Could you check a few things on this model? Use its own coordinates, in mm. Face numbers are marked on the shaded views. A direction names the side the tool comes from. Give positions to 0.01 mm unless a question says otherwise; leave off trailing zeros. Order: outer loops, then holes, each group sorted by start corner. A loop starts at its lowest first (then second) coordinate and runs counter-clockwise, first axis right, second up. Notation, with made-up numbers: M 19.5,72 L 25.5,72 A23 cw 25.5,82 Z; hole C -36,11 d10. An arc over 180 degrees is marked long. Use a Markdown table: item, result. Add a question column.
Item 1: Suppose I cut it at B-B on x = 12.7. Write out the boundary of the cut face in (y, z).
Item 2: Suppose I cut it at D-D on y = -5.75. Write out the boundary of the cut face in (x, z).
Item 3: I'm going to push flat-ended pins straight in: pin 1 Ø12 at (y, z) = (-19, 3.5) entering from -X; pin 2 Ø4 at (x, z) = (33.5, 9) entering from -Y. Where does each tip first touch, or does it pass through?
Item 4: If I drill on L1, parallel to Z at x = 12.7, y = 2.1; L2, parallel to X at y = -9, z = 2; L3, parallel to Y at x = 43.5, z = 2.5, over which ranges is the centre line in solid material (lowest first)? Write a range as from..to.
Item 5: For the marked faces 1 and 2, which set-ups out of +Z, -Z, +X, -X, +Y, -Y let a thin tool reach every point of the face, with its end or its side?
Item 6: Suppose I cut it at A-A on z = 12.7. Write out the boundary of the cut face in (x, y), plus the area to 3 significant figures.
Item 7: Suppose I cut it at C-C on z = 24.25. Write out the boundary of the cut face in (x, y).
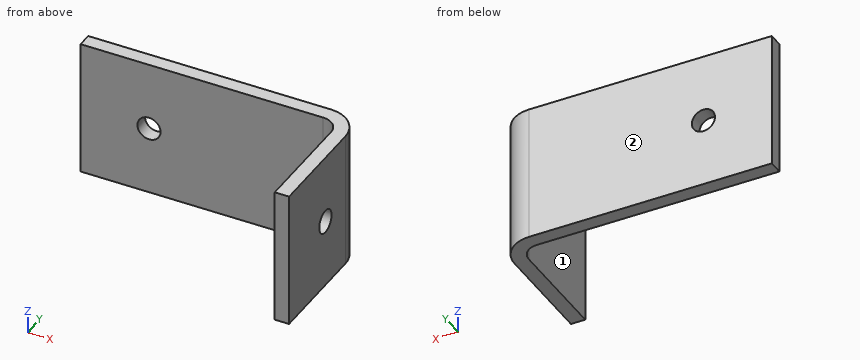
from build123d import *

# Parameters (mm, degrees)
F1_DEPTH = 25.4
F2_R     = 2.15265
F3_DEPTH = 2.65684
F4_R     = 2.15265
F5_DEPTH = 2.65684
F6_R     = 3.08356
F7_R     = 5.7404


with BuildPart() as f1:
    # F0 (on Top) → F1 (new body)
    with BuildSketch(Plane.XY):
        Polygon((0, 2.65684), (0, 0), (48.14316, 0), (48.14316, -22.74316), (50.8, -22.74316), (50.8, 2.65684), align=None)
    extrude(amount=F1_DEPTH)

    # F2 (on face) → F3 (cut, through all)
    with BuildSketch(Plane(origin=(0, 2.65684, 0), x_dir=(-1, 0, 0), z_dir=(0, 1, 0))):
        with Locations((-12.7, 12.7)):
            Circle(F2_R)
    extrude(amount=-F3_DEPTH, mode=Mode.SUBTRACT)

    # F4 (on face) → F5 (cut, through all)
    with BuildSketch(Plane.YZ.offset(50.8)):
        with Locations((-10.04316, 12.7)):
            Circle(F4_R)
    extrude(amount=-F5_DEPTH, mode=Mode.SUBTRACT)

    # F6
    f6_edges = [f1.edges().sort_by_distance(p)[0] for p in [
        (48.14316, 0, 12.7),
    ]]
    fillet(f6_edges, radius=F6_R)

    # F7
    f7_edges = [f1.edges().sort_by_distance(p)[0] for p in [
        (50.8, 2.65684, 12.7),
    ]]
    fillet(f7_edges, radius=F7_R)


solid = f1.part
Findings below:
| question | item | result |
|---|---|---|
| 1 | outline | M 0,0 L 2.66,0 L 2.66,10.55 L 0,10.55 Z; M 0,14.85 L 2.66,14.85 L 2.66,25.4 L 0,25.4 Z |
| 2 | outline | M 48.14,0 L 50.8,0 L 50.8,25.4 L 48.14,25.4 Z |
| 3 | pin 1 | stops at x = 48.14 |
| 3 | pin 2 | stops at y = 0 |
| 4 | L1 | z = 0..10.55, 14.85..25.4 |
| 4 | L2 | x = 48.14..50.8 |
| 4 | L3 | y = 0..2.66 |
| 5 | face 1 | +Z, -Z, -X, -Y |
| 5 | face 2 | +Z, -Z, +X, -X, +Y |
| 6 | outline | M 0,0 L 10.55,0 L 10.55,2.66 L 0,2.66 Z; M 14.85,0 L 45.06,0 A3.08 cw 48.14,-3.08 L 48.14,-7.89 L 50.8,-7.89 L 50.8,-3.08 A5.74 ccw 45.06,2.66 L 14.85,2.66 Z; M 48.14,-22.74 L 50.8,-22.74 L 50.8,-12.2 L 48.14,-12.2 Z |
| 6 | area | 167 mm^2 |
| 7 | outline | M 0,0 L 45.06,0 A3.08 cw 48.14,-3.08 L 48.14,-22.74 L 50.8,-22.74 L 50.8,-3.08 A5.74 ccw 45.06,2.66 L 0,2.66 Z |
